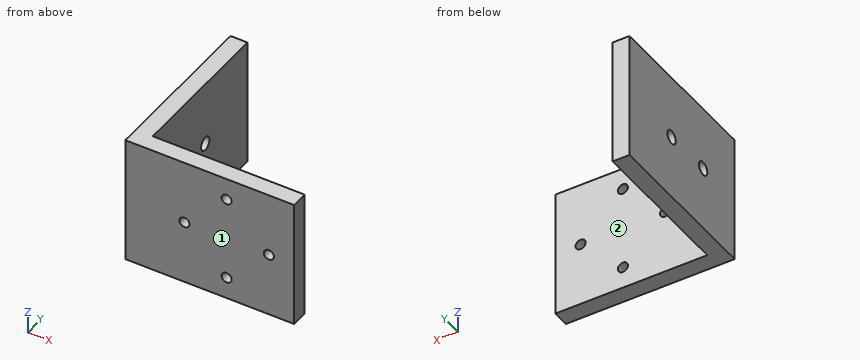
Autodesk Inventor part; units mm, degrees
ref_plane "YZ Plane" through (0, 0, 0) normal (1, 0, 0) x (0, 1, 0)
ref_plane "XZ Plane" through (0, 0, 0) normal (0, 1, 0) x (-1, 0, 0)
ref_plane "XY Plane" through (0, 0, 0) normal (0, 0, 1) x (1, 0, 0)
sketch "Sketch1" plane through (0, 0, 0) normal (0, 1, 0) x (-1, 0, 0)
  line L0 (0, 0) -> (-100, 0)
  line L1 (-100, 0) -> (-100, -76)
  line L2 (-100, -76) -> (0, -76)
  line L3 (0, -76) -> (0, 0)
  dimension "d0" = 100
  dimension "d1" = 76
extrude "Extrusion1" add sketch "Sketch1" along normal blind 10
sketch "Sketch2" plane through (0, 10, 0) normal (0, 1, 0) x (1, 0, 0)
  line L0 (0, 0) -> (100, 0)
  line L1 (100, 76) -> (0, 76)
  line L2 (0, 0) -> (10, 0)
  line L3 (10, 0) -> (10, 76)
  line L4 (10, 76) -> (0, 76)
  line L5 (0, 76) -> (0, 0)
  dimension "d4" = 10
extrude "Extrusion2" add sketch "Sketch2" along normal blind 90
sketch "Sketch3" plane through (10, 10, 0) normal (1, 0, 0) x (0, 0, -1)
  line L0 (0, -10) -> (76, -10)
  line L1 (0, -10) -> (38, -10)
  line L2 (38, -10) -> (38, 20)
  circle A0 centre (38, 20) radius 4
  line L3 (38, 20) -> (38, 50)
  circle A1 centre (38, 50) radius 4
  dimension "d7" = 30
  dimension "d8" = 8
  dimension "d9" = 30
  dimension "d10" = 8
sketch "Sketch4" plane through (0, 0, -76) normal (-1, 0, 0) x (0, 0, 1)
  circle A0 centre (38, 30) radius 4
  circle A1 centre (38, 60) radius 4
  point P0 (76, 0)
  dimension "d15" = 8
  dimension "d16" = 8
extrude "Extrusion3" cut sketch "Sketch3" against normal blind 10
sketch "Sketch5" plane through (0, 0, 0) normal (0, -1, 0) x (1, 0, 0)
  line L0 (0, -76) -> (0, 0)
  line L1 (0, -38) -> (60, -38)
  line L2 (100, 0) -> (100, -76)
  line L3 (60, -38) -> (60, -63)
  line L4 (60, -38) -> (60, -13)
  line L5 (60, -38) -> (35, -38)
  line L6 (60, -38) -> (85, -38)
  circle A0 centre (60, -63) radius 3
  circle A1 centre (85, -38) radius 3
  circle A2 centre (60, -13) radius 3
  circle A3 centre (35, -38) radius 3
  dimension "d19" = 60
  dimension "d20" = 25
  dimension "d21" = 25
  dimension "d22" = 25
  dimension "d23" = 25
  dimension "d24" = 6
  dimension "d25" = 6
  dimension "d26" = 6
  dimension "d27" = 6
extrude "Extrusion4" cut sketch "Sketch5" against normal blind 10
Model file for the job. Use its own axes, mm. Face numbers are marked on the shaded views. A direction names the side the tool comes from. Give positions to 0.01 mm unless a question says otherwise; leave off trailing zeros. Write each loop counter-clockwise with the first axis right and the second up, starting at its lowest first coordinate (ties: lowest second). Pieces come first, ordered by that corner, then holes. Notation, with made-up numbers: M 60.5,-13.75 L 73.5,-13.75 A18 ccw 73.5,-7.75 Z; hole C -25,59.25 d11. An arc over 180 degrees is marked long. Use a Markdown table: item, result.
1) Pin check, flat tips, straight feed: pin 1 (3.5 mm diameter, centred on x = 35, z = -38, fed in from -Y); pin 2 (9.5 mm diameter, centred on x = 60, z = -63, fed in from +Y); pin 3 (13 mm diameter, centred on y = 60, z = -38, fed in from +X). Stop position of each tip, or through.
Responses:
| item | result |
|---|---|
| pin 1 | passes through |
| pin 2 | stops at y = 10 |
| pin 3 | stops at x = 10 |
2) Cut at D-D (x = 60). List the corners of the cut face in (y, z), and give its area (3 significant figures).
Responses:
| item | result |
|---|---|
| outline | M 0,-76 L 10,-76 L 10,-66 L 0,-66 Z; M 0,-60 L 10,-60 L 10,-16 L 0,-16 Z; M 0,-10 L 10,-10 L 10,0 L 0,0 Z |
| area | 640 mm2 |
3) Drill centre lines: line 1 (Y direction, x = 3, z = -38); line 2 (X direction, y = 2.75, z = -38); line 3 (X direction, y = 5.5, z = -40). Where is each one in solid material? Low to high. Write a range as from..to.
Responses:
| item | result |
|---|---|
| line 1 | y = 0..26, 34..56, 64..100 |
| line 2 | x = 0..32, 38..82, 88..100 |
| line 3 | x = 0..32.76, 37.24..82.76, 87.24..100 |
4) Cut at A-A (x = 35). List the corners of the cut face in (y, z), and give its area (3 significant figures).
Responses:
| item | result |
|---|---|
| outline | M 0,-76 L 10,-76 L 10,-41 L 0,-41 Z; M 0,-35 L 10,-35 L 10,0 L 0,0 Z |
| area | 700 mm2 |
5) Cut at B-B (z = -38). List the corners of the cut face in (x, y), and give its area (3 significant figures).
Responses:
| item | result |
|---|---|
| outline | M 0,0 L 32,0 L 32,10 L 10,10 L 10,26 L 0,26 Z; M 0,34 L 10,34 L 10,56 L 0,56 Z; M 0,64 L 10,64 L 10,100 L 0,100 Z; M 38,0 L 82,0 L 82,10 L 38,10 Z; M 88,0 L 100,0 L 100,10 L 88,10 Z |
| area | 1,620 mm2 |
6) Tool access for the marked faces 1 and 2: list every direction of +Z, -Z, +X, -X, +Y, -Y with a clear straight run to the whole face (end or side of a thin tool).
Responses:
| item | result |
|---|---|
| face 1 | +Z, -Z, +X, -X, -Y |
| face 2 | +Z, -Z, +X, +Y |
7) Cut at C-C (y = 60). List the corners of the cut face in (x, z).
Responses:
| item | result |
|---|---|
| outline | M 0,-76 L 10,-76 L 10,-42 L 0,-42 Z; M 0,-34 L 10,-34 L 10,0 L 0,0 Z |
